from build123d import *

# Parameters (mm, degrees)
F0_W     = 94
F0_H     = 71
F0_W_2   = 84
F0_H_2   = 56
F1_DEPTH = 1
F2_W     = 2
F2_H     = 71
F3_DEPTH = 36
F4_R     = 1.5
F5_DEPTH = 100
F6_SIZE  = 1.87


with BuildPart() as f1:
    # F0 (on Front) → F1 (new body, symmetric)
    with BuildSketch(Plane.XZ):
        Rectangle(F0_W, F0_H)
        with Locations((0, -2.5)):
            Rectangle(F0_W_2, F0_H_2, mode=Mode.SUBTRACT)
    extrude(amount=F1_DEPTH, both=True)

    # F2 (on face) → F3 (join)
    with BuildSketch(Plane(origin=(0, 1, 0), x_dir=(-1, 0, 0), z_dir=(0, 1, 0))):
        with Locations((-46, 0)):
            Rectangle(F2_W, F2_H)
        with Locations((46, 0)):
            Rectangle(F2_W, F2_H)
    extrude(amount=F3_DEPTH)

    # F4 (on face) → F5 (cut)
    with BuildSketch(Plane(origin=(-47, 0, 0), x_dir=(0, -1, 0), z_dir=(-1, 0, 0))):
        with Locations((-30.5, -31)):
            Circle(F4_R)
        with Locations((-6.5, -31)):
            Circle(F4_R)
        with Locations((-30.5, 29)):
            Circle(F4_R)
        with Locations((-5.5, 29)):
            Circle(F4_R)
        with Locations((-30.5, 14)):
            Circle(F4_R)
        with Locations((-5.5, 14)):
            Circle(F4_R)
    extrude(amount=-F5_DEPTH, mode=Mode.SUBTRACT)

    # F6
    f6_edges = [f1.edges().sort_by_distance(p)[0] for p in [
        (-45, 32, 29),
        (-45, 32, 14),
        (-45, 7, 29),
        (45, 7, 29),
        (45, 7, 14),
        (45, 32, 29),
        (45, 32, 14),
        (-45, 7, 14),
        (45, 8, -31),
        (45, 32, -31),
        (-45, 8, -31),
        (-45, 32, -31),
    ]]
    chamfer(f6_edges, length=F6_SIZE)


solid = f1.part
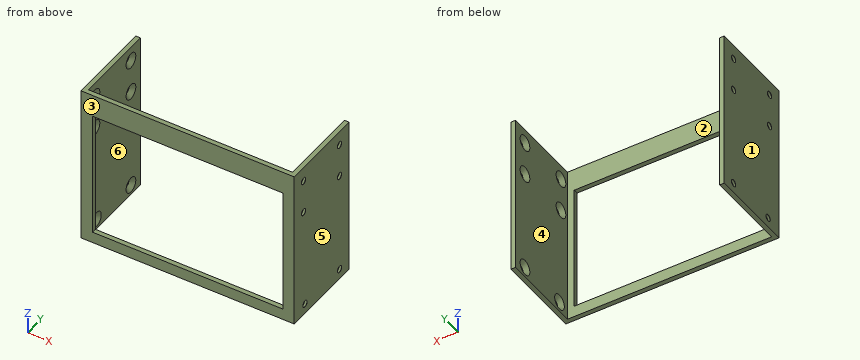
Source: CAD feature listing. Evaluate the final solid. Frame: model axes, mm. Face numbers are marked on the shaded views. A direction names the side the tool comes from. Round coordinates to 2 decimals unless told otherwise and drop trailing zeros. Write each loop counter-clockwise with the first axis right and the second up, starting at its lowest first coordinate (ties: lowest second). Pieces come first, ordered by that corner, then holes. Notation, with made-up numbers: M -16,-39 L 26,-39 A21 ccw 26,-4 Z; hole C 45.25,68.5 d9. An arc over 180 degrees is marked long. One line per item, written item: value. Start each with the question number.
Item 1: Section query A-A (y = 22.5). Return the cut outline in (x, z).
Item 2: Section query D-D (z = 29). State how many separate pieces and enclosed holes the cut face has, plus the area to 3 significant figures.
Item 3: Section query B-B (z = -20). Return the cut outline in (x, y).
Item 4: Ray query, L1, parallel to X at y = 26.5, z = -2; L2, parallel to Y at x = 46, z = 14. Return the intervals inside material, ascending. Write a range as from..to.
Item 5: Mould query, pull axis X, two halves, no side actions, for the marked faces 1, 2, 3 and 4. Classes: pulls with the +X half, pulls with the -X half, needs draft (parallel to the pull), parting line crosses it, or undercut.
Item 6: Pin query (flat end, axial travel): pin 1 (5 mm diameter, centred on y = 30.5, z = -31, fed in from +X). Return the tip coordinate at first contact, or that it passes through.
Item 7: Set-up query: the marked faces 5 and 6. Return all of +Z, -Z, +X, -X, +Y, -Y with unobstructed straight access to the full face (end or side cutting, diameter ignored); none if empty.
Item 8: Section query C-C (x = -15). Return the cut outline in (y, z).
Result set:
1. outline: M -47,-35.5 L -45,-35.5 L -45,35.5 L -47,35.5 Z; M 45,-35.5 L 47,-35.5 L 47,35.5 L 45,35.5 Z
2. separate pieces: 5
2. enclosed holes: 0
2. area: 294 mm²
3. outline: M -47,-1 L -42,-1 L -42,1 L -45,1 L -45,37 L -47,37 Z; M 42,-1 L 47,-1 L 47,37 L 45,37 L 45,1 L 42,1 Z
4. L1: x = -47..-45, 45..47
4. L2: y = -1..3.13, 7.87..28.13, 32.87..37
5. face 1: pulls with the -X half
5. face 2: undercut
5. face 3: needs draft
5. face 4: undercut
6. pin 1: stops at x = 47
7. face 5: +Z, -Z, +X, +Y, -Y
7. face 6: +Z, -Z, +Y
8. outline: M -1,-35.5 L 1,-35.5 L 1,-30.5 L -1,-30.5 Z; M -1,25.5 L 1,25.5 L 1,35.5 L -1,35.5 Z
